Can you work these out from the model? Positions are in its coordinate system, mm. Give positions to 0.01 mm unless a question says otherwise; leave off trailing zeros. Loops run counter-clockwise (first coordinate to the right, second up) from the corner with the lowest first, then second, coordinate; pieces in that order, holes last.
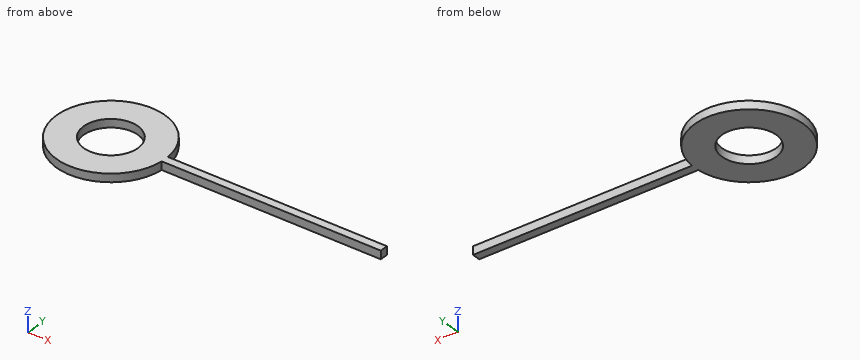
from build123d import *

# Parameters (mm, degrees)
F0_R     = 0.8382
F1_DEPTH = 0.254


with BuildPart() as f1:
    # F0 (on Top) → F1 (new body)
    with BuildSketch(Plane.XY):
        with BuildLine():
            Line((0, 0.127), (0, 0))
            Line((0, 0), (0.8333824718, 0))
            ThreePointArc((0.8333824718, 0), (0.836995185, 0.0634543302), (0.8382, 0.127))
            Line((0.8382, 0.127), (0, 0.127))
        make_face()
        with BuildLine():
            Line((0.8333824718, 0), (0, 0))
            Line((0, 0), (0, 0.127))
            Line((0, 0.127), (0, 0.254))
            Line((0, 0.254), (0.8333824718, 0.254))
            ThreePointArc((0.8333824718, 0.254), (-2.5146, 0.127), (0.8333824718, 0))
        make_face()
        with Locations((-0.8382, 0.127)):
            Circle(F0_R, mode=Mode.SUBTRACT)
        with BuildLine():
            ThreePointArc((0.8382, 0.127), (0.836995185, 0.0634543302), (0.8333824718, 0))
            Line((0.8333824718, 0), (7.62, 0))
            Line((7.62, 0), (7.62, 0.254))
            Line((7.62, 0.254), (0.8333824718, 0.254))
            ThreePointArc((0.8333824718, 0.254), (0.836995185, 0.1905456698), (0.8382, 0.127))
        make_face()
        with BuildLine():
            Line((0, 0.254), (0, 0.127))
            Line((0, 0.127), (0.8382, 0.127))
            ThreePointArc((0.8382, 0.127), (0.836995185, 0.1905456698), (0.8333824718, 0.254))
            Line((0.8333824718, 0.254), (0, 0.254))
        make_face()
    extrude(amount=F1_DEPTH)


solid = f1.part
(1) Suppose I cut it at C-C on z = 0.1. List the corners of the cut face in (x, y) for me.
Returned:
outline: (0.83, 0) - (7.62, 0) - (7.62, 0.25) - (0.83, 0.25) arc R1.68 ccw (long way) to start; hole circle Ø1.68 at (-0.84, 0.13)
(2) Suppose I cut it at D-D on x = 6.25. List the corners of the cut face in (y, z) for me.
Returned:
outline: (0, 0) - (0.25, 0) - (0.25, 0.25) - (0, 0.25) - close
(3) Suppose I cut it at B-B on x = -0.5. List the corners of the cut face in (y, z) for me.
Returned:
outline: (-1.51, 0) - (-0.64, 0) - (-0.64, 0.25) - (-1.51, 0.25) - close; (0.89, 0) - (1.77, 0) - (1.77, 0.25) - (0.89, 0.25) - close
(4) Suppose I cut it at A-A on y = -0.1. List the corners of the cut face in (x, z) for me.
Returned:
outline: (-2.5, 0) - (-1.65, 0) - (-1.65, 0.25) - (-2.5, 0.25) - close; (-0.03, 0) - (0.82, 0) - (0.82, 0.25) - (-0.03, 0.25) - close
(5) Please list where these lines run through material, in increasing order: probe 1 along X at (y, z) = (0.1, 0.1); probe 2 along Y at (x, z) = (4.5, 0.2); probe 3 along X at (y, z) = (-0.55, 0.1).
Returned:
probe 1: x = -2.51 to -1.68, 0 to 7.62
probe 2: y = 0 to 0.25
probe 3: x = -2.37 to -1.33, -0.34 to 0.7
